Can you work these out from the drawing? Everything is in mm from the part's minimum corner. A direction names the side the tool comes from. Give positions to 0.01 mm unless a question says otherwise; leave off trailing zeros. Write each loop counter-clockwise with the first axis right and the second up, starting at its lowest first coordinate (ties: lowest second). Pieces come first, ordered by that corner, then holes. Notation, with made-up numbers: M 46,-30 L 89,-30 A3 ccw 89,-26 Z; hole C 17.5,38 d2. An arc over 180 degrees is marked long. One line per item, written item: value.
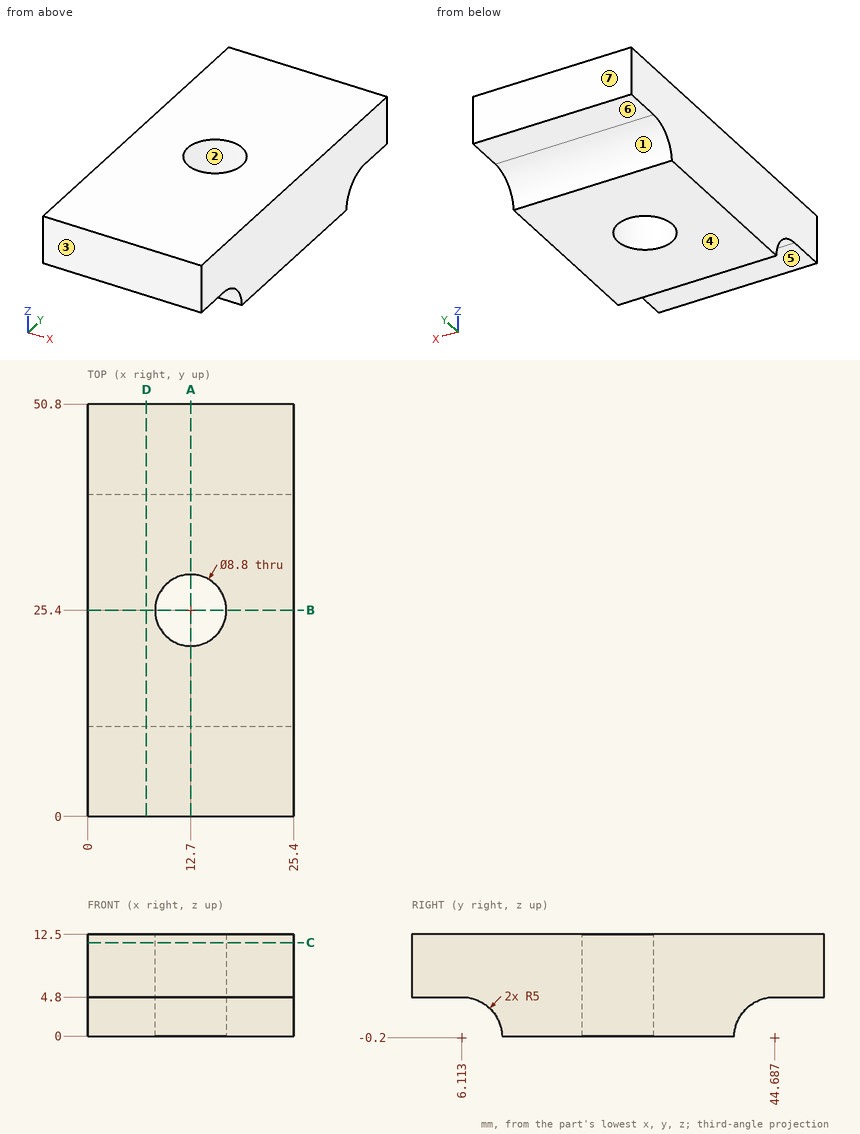
1) If we section it at D-D, the plane x = 7.25: Write out the boundary of the cut face in (y, z).
Outcome:
outline: M 0,4.8 L 6.11,4.8 A5 cw 11.11,0 L 39.69,0 A5 cw 44.69,4.8 L 50.8,4.8 L 50.8,12.5 L 0,12.5 Z
2) We'd pull the mould along Y, two halves only. Please class the marked faces 1, 2, 3 and 4: pulls with the +Y half, pulls with the -Y half, needs draft (parallel to the pull), parting line crosses it, or undercut.
Outcome:
face 1: pulls with the +Y half
face 2: undercut
face 3: pulls with the -Y half
face 4: needs draft
3) I'm going to push flat-ended pins straight in: pin 1 (1 mm diameter, centred on x = 19, z = 2, fed in from +Y); pin 2 (1.8 mm diameter, centred on x = 7, y = 2.5, fed in from -Z). Where does each tip first touch, or does it pass through?
Outcome:
pin 1: stops at y = 40.48
pin 2: stops at z = 4.8
4) On a 3-axis mill with a long thin cutter (end or side, diameter ignored), from which of +Z, -Z, +X, -X, +Y, -Y can I reach the whole of each face in a straight line? I mean the marked faces 5, 6 and 7. Say none if no direction works.
Outcome:
face 5: -Z, +X, -X, -Y
face 6: -Z, +X, -X, +Y
face 7: +Z, -Z, +X, -X, +Y
5) If we section it at A-A, the plane x = 12.7: Write out the boundary of the cut face in (y, z), then the cut area to 3 significant figures.
Outcome:
outline: M 0,4.8 L 6.11,4.8 A5 cw 11.11,0 L 21,0 L 21,12.5 L 0,12.5 Z; M 29.8,0 L 39.69,0 A5 cw 44.69,4.8 L 50.8,4.8 L 50.8,12.5 L 29.8,12.5 Z
area: 429 mm^2
6) If we section it at B-B, the plane y = 25.4: Write out the boundary of the cut face in (x, z).
Outcome:
outline: M 0,0 L 8.3,0 L 8.3,12.5 L 0,12.5 Z; M 17.1,0 L 25.4,0 L 25.4,12.5 L 17.1,12.5 Z
7) If we section it at C-C, the plane z = 11.5: Write out the boundary of the cut face in (x, y).
Outcome:
outline: M 0,0 L 25.4,0 L 25.4,50.8 L 0,50.8 Z; hole C 12.7,25.4 d8.8
8) Please list where these lines run through material, in increasing order: L1, parallel to Y at x = 12.7, z = 7.25; L2, parallel to X at y = 22, z = 9.25 (1 decimal); L3, parallel to Y at x = 12, z = 5.25 (1 decimal). Write a range as from..to.
Outcome:
L1: y = 0..21, 29.8..50.8
L2: x = 0..9.9, 15.5..25.4
L3: y = 0..21.1, 29.7..50.8
